Autodesk Fusion 360 part; units mm, degrees
sketch "Sketch1" plane through (0, 0, 0) normal (0, 0, 1) x (1, 0, 0)
  line L0 (0, 0) -> (57.1, 0)
  line L1 (57.1, 0) -> (57.1, 152.3)
  line L2 (57.1, 152.3) -> (0, 152.3)
  line L3 (0, 152.3) -> (0, 0)
  circle A0 centre (28.5, 4) radius 1.2512
  circle A1 centre (52.5, 148) radius 1.2512
  circle A2 centre (4.5, 148) radius 1.2512
  line L4 (6, 69) -> (11, 69)
  line L5 (11, 69) -> (11, 1)
  line L6 (11, 1) -> (6, 1)
  line L7 (6, 1) -> (6, 69)
  line L8 (46, 1) -> (46, 69)
  line L9 (46, 69) -> (51, 69)
  line L10 (51, 69) -> (51, 1)
  line L11 (51, 1) -> (46, 1)
  line L12 (15, 121) -> (27, 121)
  line L13 (27, 121) -> (27, 109)
  line L14 (27, 109) -> (15, 109)
  line L15 (15, 109) -> (15, 121)
  line L16 (48.19, 128.3216) -> (56.4181, 128.3216)
  line L17 (56.4181, 128.3216) -> (56.4181, 124.9122)
  line L18 (56.4181, 124.9122) -> (48.19, 124.9122)
  line L19 (48.19, 124.9122) -> (48.19, 128.3216)
  line L20 (22.55, 151.4) -> (34.55, 151.4)
  line L21 (34.55, 151.4) -> (34.55, 141.4)
  line L22 (34.55, 141.4) -> (22.55, 141.4)
  line L23 (22.55, 141.4) -> (22.55, 151.4)
  dimension "d1" = 57.1
  dimension "d2" = 152.3
  dimension "d6" = 5
  dimension "d7" = 68
  dimension "d8" = 5
  dimension "d9" = 68
  dimension "d10" = 12
  dimension "d13" = 12
  dimension "d14" = 10
extrude "Extrude1" add sketch "Sketch1" against normal blind 2.5 contours L8 L9 L10 L11 makes body 1
extrude "Extrude2" add sketch "Sketch1" against normal blind 2.5 separate body contours L4 L5 L6 L7 makes body 2
extrude "Extrude3" add sketch "Sketch1" against normal blind 2.5 separate body contours L12 L13 L14 L15 makes body 3
extrude "Extrude4" add sketch "Sketch1" against normal blind 2.5 separate body contours L16 L17 L18 L19 makes body 4
extrude "Extrude5" add sketch "Sketch1" against normal blind 2.5 separate body contours L20 L21 L22 L23 makes body 5
extrude "Extrude6" add sketch "Sketch1" against normal blind 4 bodies 1 2 3 4 5
extrude "Extrude7" add 1 faces at (28.5262, 47.7496, -4) along direction (0, 0, -1) blind 1.2 on bodies 1 bodies 1
extrude "Extrude8" add 1 faces at (19.0333, 152.3, -3.4667) along direction (0, 1, 0) blind 0.25 on bodies 1 bodies 1
fillet "Fillet5" radius 6 4 edges at (57.1, 0, -2.6) (0, 0, -2.6) (0, 152.55, -2.6) (57.1, 152.55, -2.6) on bodies 1
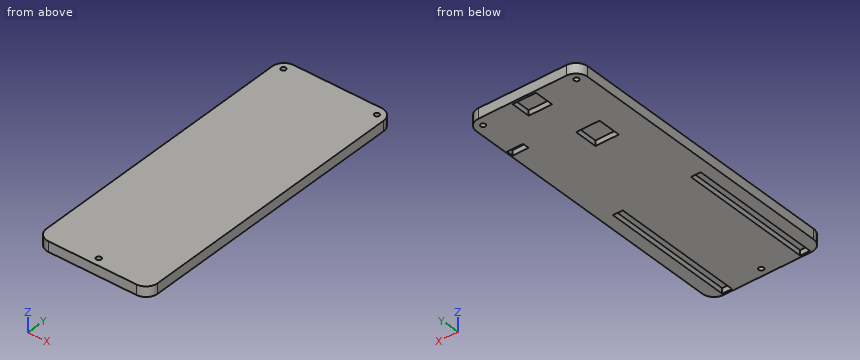
Could you check a few things on this model? Use its own coordinates, in mm. Coordinates: 2 decimals unless noted, no trailing zeros. Order: outer loops, then holes, each group sorted by start corner. A loop starts at its lowest first (then second) coordinate and runs counter-clockwise, first axis right, second up. Notation, with made-up numbers: M 69.25,50 L 82.25,50 A27 cw 82.25,84 Z; hole C 3,-12.5 d3. An arc over 180 degrees is marked long. Use one line per item in the form item = value. Start each with the question number.
1. For pin 1 (0.8 mm diameter, centred on x = 52.5, z = -4, fed in from -Y); pin 2 (1.4 mm diameter, centred on y = 147, z = -4.5, fed in from +X); pin 3 (6 mm diameter, centred on x = 20.5, y = 115.5, fed in from -Z); pin 4 (1.5 mm diameter, centred on x = 28.5, y = 4, fed in from -Z), each with a flat end and sliding along its axis, tell me the tip position at first contact or that it passes through.
2. Suppose I cut it at A-A on z = -4.4. Count the separate pieces of the cut face and the enclosed holes in it, then the cut area to 3 significant figures.
3. Please list where these lines run through material, in increasing order: line 1 (X direction, y = 25.5, z = -2.55); line 2 (X direction, y = 126.5, z = -2.7); line 3 (Y direction, x = 28.5, z = -2.25).
4. Suppose I cut it at C-C on x = 25. Write out the boundary of the cut face in (y, z), then the cut area to 3 significant figures.
5. Suppose I cut it at B-B on y = 116. Write out the boundary of the cut face in (x, z), then the cut area to 3 significant figures.
6. Suppose I cut it at D-D on y = 39. Write out the boundary of the cut face in (x, z), then the cut area to 3 significant figures.
Geometry says:
q1.pin_1 = 0.08
q1.pin_2 = 57.1
q1.pin_3 = -2.5
q1.pin_4 = through
q2.separate_pieces = 1
q2.enclosed_holes = 8
q2.area = 7,690 mm^2
q3.line_1 = 0 to 6, 11 to 46, 51 to 57.1
q3.line_2 = 0 to 48.19, 56.42 to 57.1
q3.line_3 = 0 to 2.75, 5.25 to 152.55
q4.outline = M 0,-5.2 L 109,-5.2 L 109,-2.5 L 121,-2.5 L 121,-5.2 L 141.4,-5.2 L 141.4,-2.5 L 151.4,-2.5 L 151.4,-5.2 L 152.55,-5.2 L 152.55,0 L 0,0 Z
q4.area = 734 mm^2
q5.outline = M 0,-5.2 L 15,-5.2 L 15,-2.5 L 27,-2.5 L 27,-5.2 L 57.1,-5.2 L 57.1,0 L 0,0 Z
q5.area = 265 mm^2
q6.outline = M 0,-5.2 L 6,-5.2 L 6,-2.5 L 11,-2.5 L 11,-5.2 L 46,-5.2 L 46,-2.5 L 51,-2.5 L 51,-5.2 L 57.1,-5.2 L 57.1,0 L 0,0 Z
q6.area = 270 mm^2
